Can you work these out from the model? Positions are in its coordinate system, mm. A direction names the side the tool comes from. Give positions to 0.01 mm unless a question says otherwise; leave off trailing zeros. Order: outer loops, then holes, each group sorted by start corner. A loop starts at its lowest first (then second) coordinate and runs counter-clockwise, first axis right, second up. Notation, with made-up numbers: (-13, 60.25) -> (11, 60.25) arc R18 cw to (11, 95.25) -> close; hole circle Ø5 at (35, 72.25). An arc over 180 degrees is marked (long way). Answer as a JSON object with one key per item and string values.
```python
from build123d import *

# Parameters (mm, degrees)
BOSS_EXTRUDE1_DEPTH = 4.5
FILLET1_R           = 13


with BuildPart() as part:
    # Sketch1 → Boss-Extrude1 (new body)
    with BuildSketch(Plane(origin=(0, 0, 0), x_dir=(1, 0, 0), z_dir=(0, 1, 0))):
        Polygon((110.219806784, 25), (110.219806784, 50), (12.469806784, 50), (12.469806784, 37.5), (7.969806784, 37.5), (7.969806784, 50), (-89.780193216, 50), (-89.780193216, 25), (10.219806784, 0), align=None)
    extrude(amount=BOSS_EXTRUDE1_DEPTH)

    # Fillet1
    fillet1_edges = [part.edges().sort_by_distance(p)[0] for p in [
        (110.219806784, 2.25, -50),
        (110.219806784, 2.25, -25),
        (-89.780193216, 2.25, -25),
        (-89.780193216, 2.25, -50),
    ]]
    fillet(fillet1_edges, radius=FILLET1_R)


solid = part.part
```
1. If we mould it in two halves opening along X, with no side actions, what happens to faces 3 (the face through (10, 2, -37.5)), 4 (the face through (106.513, 2.282, -46.091)), 5 (the face through (-87.101, 2.282, -27.245))? For each: +X half, -X half, draft (parallel to the pull), parting line (faces both ways), or undercut.
Worked answers:
{"face 3": "undercut", "face 4": "+X half", "face 5": "-X half"}
2. For faces 1 (the face through (12.47, 2, -44)), 2 (the face through (-35.488, 2.218, -11.427)), which set-ups out of +Z, -Z, +X, -X, +Y, -Y let a thin tool reach every point of the face, with its end or its side?
Worked answers:
{"face 1": "-Z, +Y, -Y", "face 2": "+Z, -X, +Y, -Y"}
3. If we section it at C-C on x = 4: Please give me the cut outline in (y, z), then the cut area to 3 significant figures.
Worked answers:
{"outline": "(0, -50) -> (4.5, -50) -> (4.5, -1.55) -> (0, -1.55) -> close", "area": "218 mm²"}
4. If we section it at B-B on z = -43: Please give me the cut outline in (x, y), then the cut area to 3 significant figures.
Worked answers:
{"outline": "(-88.31, 0) -> (7.97, 0) -> (7.97, 4.5) -> (-88.31, 4.5) -> close; (12.47, 0) -> (108.75, 0) -> (108.75, 4.5) -> (12.47, 4.5) -> close", "area": "867 mm²"}
5. Will these pins go through, and if not, where does the flat tip stop? pin 1 Ø1.3 at (x, y) = (10.5, 2) entering from -Z; pin 2 Ø1.3 at (y, z) = (3.5, -41.5) entering from -X; pin 3 Ø1.3 at (y, z) = (3, -44.5) entering from +X.
Worked answers:
{"pin 1": "z = -37.5", "pin 2": "x = -89.2", "pin 3": "x = 108.27"}
6. If we section it at D-D on z = -17.5: Please give me the cut outline in (x, y), then the cut area to 3 significant figures.
Worked answers:
{"outline": "(-59.78, 0) -> (80.22, 0) -> (80.22, 4.5) -> (-59.78, 4.5) -> close", "area": "630 mm²"}
7. If we section it at A-A on y = 2.9: Please give me the cut outline in (x, z).
Worked answers:
{"outline": "(-89.78, -37) arc R13 ccw to (-76.78, -50) -> (7.97, -50) -> (7.97, -37.5) -> (12.47, -37.5) -> (12.47, -50) -> (97.22, -50) arc R13 ccw to (110.22, -37) -> (110.22, -35.15) arc R13 ccw to (100.37, -22.54) -> (10.22, 0) -> (-79.93, -22.54) arc R13 ccw to (-89.78, -35.15) -> close"}
8. Please list where these lines run through material, in increasing order: L1, parallel to X at y = 2.05, z = -35; L2, parallel to X at y = 0.65, z = -44; L3, parallel to Z at x = 87.5, y = 0.6.
Worked answers:
{"L1": "-89.78 to 110.22", "L2": "-87.73 to 7.97, 12.47 to 108.17", "L3": "-50 to -19.32"}
